Answer from the drawing. Dimensions are ordinates in mm from the lowest x, y and z of the part. A direction names the side the tool comes from. Round coordinates to 2 decimals unless told otherwise and drop trailing zeros. Write each loop counter-clockwise with the first axis right and the second up, starting at its lowest first coordinate (ties: lowest second). Pieces come first, ordered by that corner, then holes. Notation, with made-up numbers: (-8.5, 30.25) - (1.5, 30.25) arc R29 cw to (1.5, 61.25) - close; hole circle Ø2 at (8.25, 16). An arc over 180 degrees is marked (long way). One line per item, written item: value. Start each with the question number.
(1) For the marked faces 5, 6 and 7, determine the directions among +Z, -Z, +X, -X, +Y, -Y from which every point of the face is accessible in a straight line to the end or side of a thin tool.
(2) A cutting plane is placed at A-A, the plane z = 8.1. Determine the outline of the cut face in (x, y) (3 decimals).
(3) Flat-ended cylindrical pins translate along their axes: pin 1 Ø2.5 at (x, z) = (3.5, 9.5) entering from -Y; pin 2 Ø1.5 at (x, z) = (23.5, 9.5) entering from +Y; pin 3 Ø2 at (x, y) = (27.5, 6.5) entering from -Z; pin 4 Ø3 at (x, z) = (7, 10.5) entering from -Y. Find the tip coordinate at first contact, or state that the pin passes through.
(4) Find the intervals of material crossed by L1, parallel to X at y = 5.55, z = 8.1 (3 decimals); L2, parallel to Z at x = 7, y = 2.5; L3, parallel to X at y = 3, z = 2, in increasing order.
(5) A cutting plane is placed at B-B, the plane x = 21.9. Determine the outline of the cut face in (y, z), plus the area to 3 significant figures.
(6) A cutting plane is placed at D-D, the plane x = 2.65. Determine the outline of the cut face in (y, z) (3 decimals).
(7) A cutting plane is placed at C-C, the plane y = 1.5. Determine the outline of the cut face in (x, z), plus the area to 3 significant figures.
(8) The mould has two halves that part along Z. Classify the marked faces 1, 2, 3 and 4: +Z half, -Z half, draft (parallel to the pull), parting line (faces both ways), or undercut.
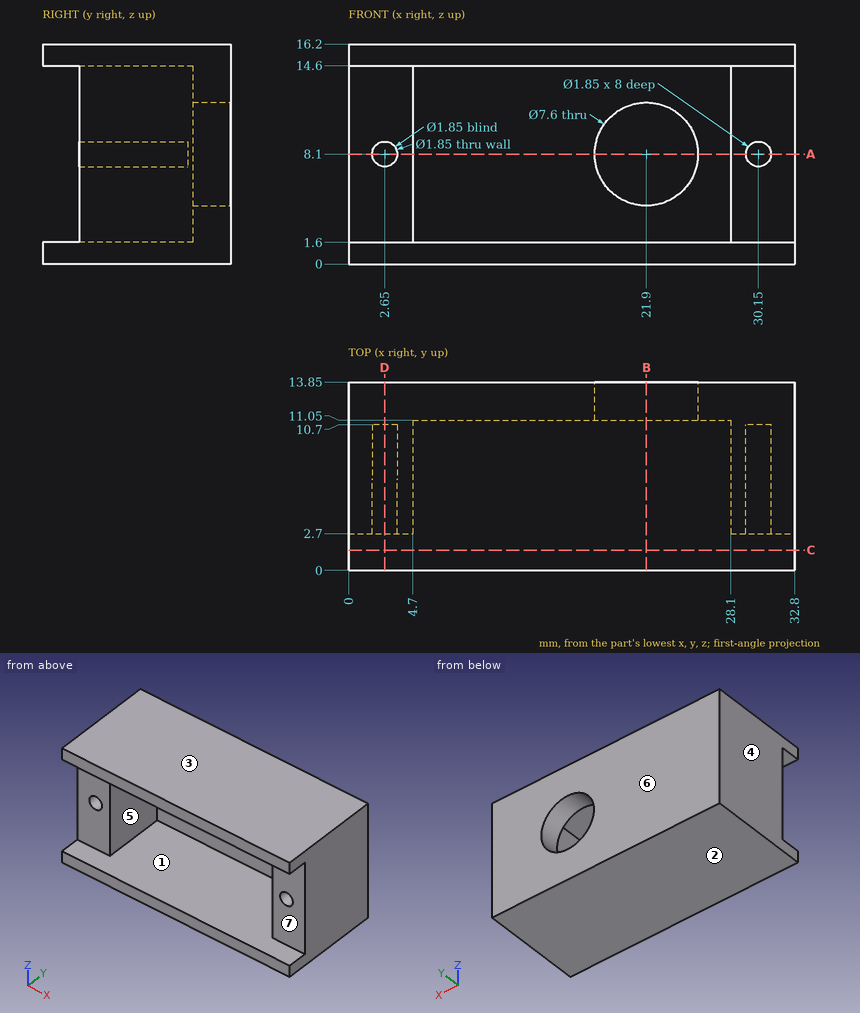
Here are the results:
1. face 5: -Y
1. face 6: +Z, -Z, +X, -X, +Y
1. face 7: +X, -X, -Y
2. outline: (0, 2.7) - (1.725, 2.7) - (1.725, 10.7) - (3.575, 10.7) - (3.575, 2.7) - (4.7, 2.7) - (4.7, 11.05) - (18.1, 11.05) - (18.1, 13.85) - (0, 13.85) - close; (25.7, 11.05) - (28.1, 11.05) - (28.1, 2.7) - (29.225, 2.7) - (29.225, 10.7) - (31.075, 10.7) - (31.075, 2.7) - (32.8, 2.7) - (32.8, 13.85) - (25.7, 13.85) - close
3. pin 1: y = 2.7
3. pin 2: through
3. pin 3: z = 0
3. pin 4: y = 11.05
4. L1: 0 to 1.725, 3.575 to 4.7, 28.1 to 29.225, 31.075 to 32.8
4. L2: 0 to 1.6, 14.6 to 16.2
4. L3: 0 to 4.7, 28.1 to 32.8
5. outline: (0, 0) - (13.85, 0) - (13.85, 4.3) - (11.05, 4.3) - (11.05, 1.6) - (0, 1.6) - close; (0, 14.6) - (11.05, 14.6) - (11.05, 11.9) - (13.85, 11.9) - (13.85, 16.2) - (0, 16.2) - close
5. area: 59.4 mm²
6. outline: (0, 0) - (13.85, 0) - (13.85, 16.2) - (0, 16.2) - (0, 14.6) - (2.7, 14.6) - (2.7, 9.025) - (10.7, 9.025) - (10.7, 7.175) - (2.7, 7.175) - (2.7, 1.6) - (0, 1.6) - close
7. outline: (0, 0) - (32.8, 0) - (32.8, 1.6) - (0, 1.6) - close; (0, 14.6) - (32.8, 14.6) - (32.8, 16.2) - (0, 16.2) - close
7. area: 105 mm²
8. face 1: undercut
8. face 2: -Z half
8. face 3: +Z half
8. face 4: draft
